```python
from build123d import *

# Parameters (mm, degrees)
CSK_FOR_3_8_FLAT_HEAD_MACHINE_SCREW_100_D           = 10.0838
CSK_FOR_3_8_FLAT_HEAD_MACHINE_SCREW_100_DEPTH       = 25.4
CSK_FOR_3_8_FLAT_HEAD_MACHINE_SCREW_100_CSINK_D     = 19.3548
CSK_FOR_3_8_FLAT_HEAD_MACHINE_SCREW_100_CSINK_ANGLE = 100
CSK_FOR_3_8_FLAT_HEAD_MACHINE_SCREW_100_TIP         = 3.029479155
FILLET1_R                                           = 2.54
CHAMFER1_SIZE                                       = 2.54
SKETCH4_R                                           = 27.94
SKETCH4_R_2                                         = 25.4
BOSS_EXTRUDE1_DEPTH                                 = 2.54
CUT_EXTRUDE1_START                                  = -508
SKETCH5_R                                           = 25.4
CUT_EXTRUDE1_DEPTH                                  = 508


with BuildPart() as part:
    # Sketch1 → Revolve1 (revolve)
    with BuildSketch(Plane.XY):
        Polygon((0, 0), (0, 15.24), (27.305, 15.24), (27.305, 23.876), (57.15, 23.876), (57.15, 49.2125), (1103.122, 49.2125), (1103.122, 50.8), (1115.822, 50.8), (1115.822, 0), align=None)
    revolve(axis=Axis((1115.822, 0, 0), (-1, 0, 0)))

    # CSK for 3/8 Flat Head Machine Screw (100)1
    with Locations(Plane.ZY):
        with Locations((0, 0)):
            CounterSinkHole(CSK_FOR_3_8_FLAT_HEAD_MACHINE_SCREW_100_D / 2, CSK_FOR_3_8_FLAT_HEAD_MACHINE_SCREW_100_CSINK_D / 2, depth=CSK_FOR_3_8_FLAT_HEAD_MACHINE_SCREW_100_DEPTH, counter_sink_angle=CSK_FOR_3_8_FLAT_HEAD_MACHINE_SCREW_100_CSINK_ANGLE)
            with Locations((0, 0, -(CSK_FOR_3_8_FLAT_HEAD_MACHINE_SCREW_100_DEPTH + CSK_FOR_3_8_FLAT_HEAD_MACHINE_SCREW_100_TIP / 2))):  # 118° drill point
                Cone(0, CSK_FOR_3_8_FLAT_HEAD_MACHINE_SCREW_100_D / 2, CSK_FOR_3_8_FLAT_HEAD_MACHINE_SCREW_100_TIP, mode=Mode.SUBTRACT)

    # Fillet1
    fillet1_edges = [part.edges().sort_by_distance(p)[0] for p in [
        (0, -15.24, 0),
    ]]
    fillet(fillet1_edges, radius=FILLET1_R)

    # Chamfer1
    chamfer1_edges = [part.edges().sort_by_distance(p)[0] for p in [
        (27.305, -23.876, 0),
    ]]
    chamfer(chamfer1_edges, length=CHAMFER1_SIZE)

    # Sketch4 → Boss-Extrude1 (add)
    with BuildSketch(Plane(origin=(1115.822, 0, 0), x_dir=(0, 0, -1), z_dir=(1, 0, 0))):
        with Locations(Location((0, 0, 0), (0, 0, 90))):
            Circle(SKETCH4_R)
        with Locations(Location((0, 0, 0), (0, 0, 90))):
            Circle(SKETCH4_R_2, mode=Mode.SUBTRACT)
    extrude(amount=BOSS_EXTRUDE1_DEPTH)

    # Sketch5 → Cut-Extrude1 (cut)
    with BuildSketch(Plane(origin=(1118.362, 0, 0), x_dir=(0, 0, -1), z_dir=(1, 0, 0)).offset(CUT_EXTRUDE1_START)):
        with Locations(Location((0, 0, 0), (0, 0, 90))):
            Circle(SKETCH5_R)
    extrude(amount=CUT_EXTRUDE1_DEPTH, mode=Mode.SUBTRACT)


solid = part.part
```
The listing builds one solid part. Answer for the finished solid, in the listing's coordinates (mm). A direction names the side the tool comes from. Give positions to 0.01 mm unless a question says otherwise; leave off trailing zeros. Order: outer loops, then holes, each group sorted by start corner. A loop starts at its lowest first (then second) coordinate and runs counter-clockwise, first axis right, second up. Notation, with made-up numbers: (28, 70) -> (87, 70) arc R28 cw to (87, 91) -> close; hole circle Ø6 at (75.5, 76.25). An arc over 180 degrees is marked (long way). One line per item, written item: value.
1) Find the intervals of material crossed by line 1 (Z direction, x = 966, y = 0); line 2 (Z direction, x = 19.75, y = 0), in increasing order.
Reported:
line 1: z = -49.21 to -25.4, 25.4 to 49.21
line 2: z = -15.24 to -5.04, 5.04 to 15.24
2) Find section B-B, the plane x = 391. Determine the outline of the cut face in (y, z) (1 decimal).
Reported:
outline: circle Ø98.4 at (0, 0)
3) A tool of negligible diameter and unlimited length cuts with its end or side. For faces 1 (the flat face through (1103.122, 27, -42)), 2 (the cylindrical face through (1109.561, -11.012, 49.592)), 3 (the flat face through (610.362, 0, 0)), from which of +Z, -Z, +X, -X, +Y, -Y can it reach the whole face along a straight path? Write none if from no direction.
Reported:
face 1: -X
face 2: +X, -X
face 3: +X
4) Flat-ended cylindrical pins translate along their axes: P1, Ø8, axis at x = 167.5, y = 30.5, coming from the -Z side; P2, Ø12, axis at x = 232, z = -34, coming from the -Y side; P3, Ø2, axis at y = -40, z = 0.5, coming from the -X side. Find the tip coordinate at first contact, or state that the pin passes through.
Reported:
P1: stops at z = -41.47
P2: stops at y = -40.47
P3: stops at x = 57.15
5) Find section A-A, the plane x = 671. Determine the outline of the cut face in (y, z) (1 decimal), plus the area to 3 significant figures.
Reported:
outline: circle Ø98.4 at (0, 0); hole circle Ø50.8 at (0, 0)
area: 5,580 mm^2
